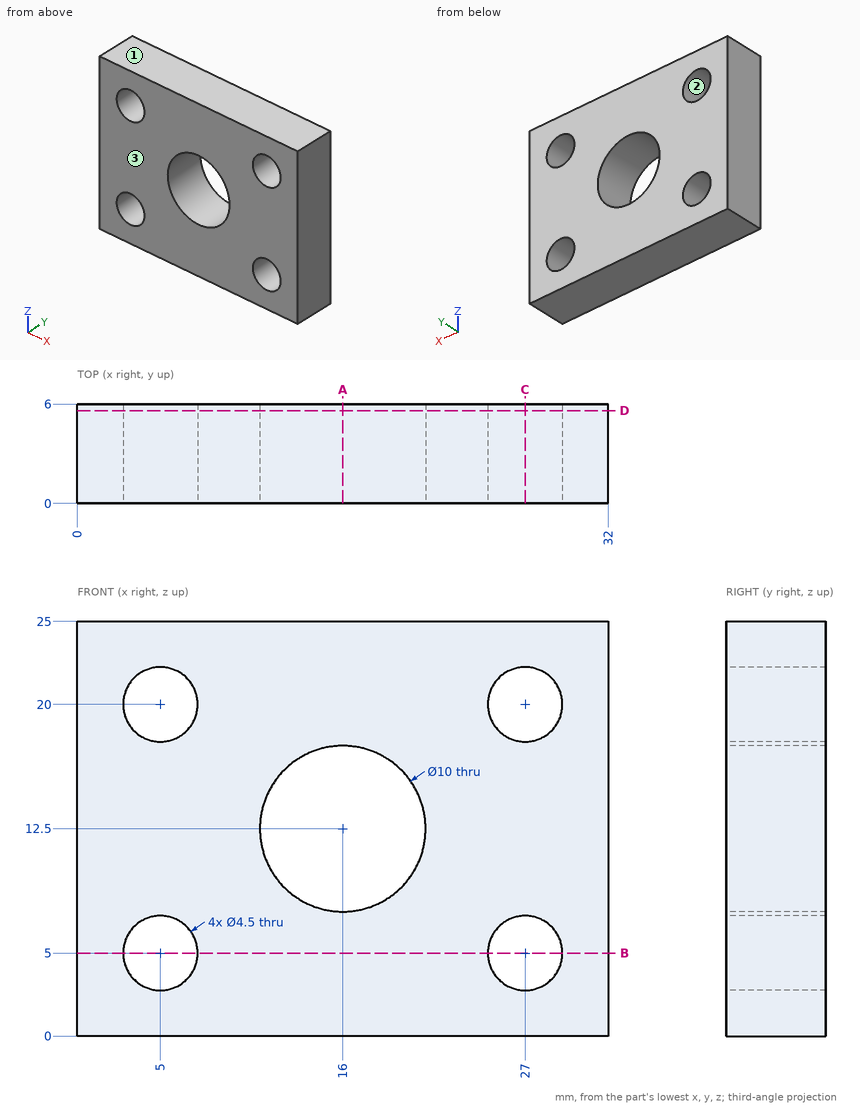
Study the drawing (mm; zero at the part's minimum x, y, z) and answer. Give positions to 0.01 mm unless a question says otherwise; leave off trailing zeros. Loops run counter-clockwise (first coordinate to the right, second up) from the corner with the lowest first, then second, coordinate; pieces in that order, holes last. Notation, with made-up numbers: M 65.5,39.5 L 77.5,39.5 A28 cw 77.5,76.5 Z; hole C 34,64 d7. An arc over 180 degrees is marked long. Use CSV: the item, a comma, the result in double quotes.
1) Find section C-C on x = 27. Write down the section's boundary in (y, z).
Answer:
outline,"M 0,0 L 6,0 L 6,2.75 L 0,2.75 Z; M 0,7.25 L 6,7.25 L 6,17.75 L 0,17.75 Z; M 0,22.25 L 6,22.25 L 6,25 L 0,25 Z"
2) Find section D-D on y = 5.6. Write down the section's boundary in (x, z), plus the area to 3 significant figures.
Answer:
outline,"M 0,0 L 32,0 L 32,25 L 0,25 Z; hole C 5,5 d4.5; hole C 5,20 d4.5; hole C 16,12.5 d10; hole C 27,5 d4.5; hole C 27,20 d4.5"
area,"658 mm^2"
3) Determine the mould class of the marked faces 1, 2 and 3 for opening direction Z: released by +Z, released by -Z, zero draft, split by the parting line, or undercut.
Answer:
face 1,"released by +Z"
face 2,"undercut"
face 3,"zero draft"
4) Find section B-B on z = 5. Write down the section's boundary in (x, y), plus the area to 3 significant figures.
Answer:
outline,"M 0,0 L 2.75,0 L 2.75,6 L 0,6 Z; M 7.25,0 L 24.75,0 L 24.75,6 L 7.25,6 Z; M 29.25,0 L 32,0 L 32,6 L 29.25,6 Z"
area,"138 mm^2"
5) Consider L1, parallel to X at y = 1.3, z = 20; L2, parallel to Z at x = 5, y = 4.7; L3, parallel to Z at x = 4, y = 3.7. Determine where each line is inside the solid, lowest interval first.
Answer:
L1,"0 to 2.75, 7.25 to 24.75, 29.25 to 32"
L2,"0 to 2.75, 7.25 to 17.75, 22.25 to 25"
L3,"0 to 2.98, 7.02 to 17.98, 22.02 to 25"
6) Find section A-A on x = 16. Write down the section's boundary in (y, z), plus the area to 3 significant figures.
Answer:
outline,"M 0,0 L 6,0 L 6,7.5 L 0,7.5 Z; M 0,17.5 L 6,17.5 L 6,25 L 0,25 Z"
area,"90.0 mm^2"
